```python
from build123d import *

# Parameters (mm, degrees)
SKETCH_1_W               = 23
SKETCH_1_H               = 27.6
SKETCH_1_W_2             = 4.5
SKETCH_1_H_2             = 1.2
EXTRUDE_1_DEPTH          = 6
SKETCH_2_R               = 4.2
EXTRUDE_2_DEPTH          = 0.85
CHAMFER_1_SIZE           = 0.3
SKETCH_4_R               = 2.5
SKETCH_4_R_2             = 1
EXTRUDE_3_DEPTH          = 3
CUT_EXTRUDE_1_DEPTH      = 28.699097458
CUT_EXTRUDE_1_DEPTH_BACK = 28.699097458
SKETCH_3_R               = 1.25
FILLET_1_R               = 1
SKETCH_5_W               = 5.6
SKETCH_5_H               = 3.5
EXTRUDE_4_DEPTH          = 3.5
SKETCH_6_R               = 0.6
EXTRUDE_7_DEPTH          = 6.5


with BuildPart() as part:
    # Эскиз1 → Бобышка-Вытянуть1 (new, symmetric)
    with BuildSketch(Plane.XY):
        Rectangle(SKETCH_1_W, SKETCH_1_H)
        with Locations((-13.75, 7.4)):
            Rectangle(SKETCH_1_W_2, SKETCH_1_H_2)
        with Locations((13.75, 7.4)):
            Rectangle(SKETCH_1_W_2, SKETCH_1_H_2)
    extrude(amount=EXTRUDE_1_DEPTH, both=True)

    # Эскиз2 → Бобышка-Вытянуть2 (add)
    with BuildSketch(Plane(origin=(0, 13.8, 0), x_dir=(1, 0, 0), z_dir=(0, 1, 0))):
        with Locations(Location((-5.8, 0, 0), (0, 0, 270))):
            Circle(SKETCH_2_R)
    extrude(amount=EXTRUDE_2_DEPTH)

    # Фаска1
    chamfer_1_edges = [part.edges().sort_by_distance(p)[0] for p in [
        (-5.8, 14.65, -4.2),
    ]]
    chamfer(chamfer_1_edges, length=CHAMFER_1_SIZE)

    # Эскиз4 → Бобышка-Вытянуть3 (add)
    with BuildSketch(Plane(origin=(0, 14.65, 0), x_dir=(1, 0, 0), z_dir=(0, 1, 0))):
        with Locations(Location((-5.8, 0, 0), (0, 0, 270))):
            Circle(SKETCH_4_R)
        with Locations(Location((-5.8, 0, 0), (0, 0, 270))):
            Circle(SKETCH_4_R_2, mode=Mode.SUBTRACT)
    extrude(amount=EXTRUDE_3_DEPTH)

    # Эскиз3 → Вырез-Вытянуть1 (cut, two sides: drawn at the far end of the back side and taken through both)
    with BuildSketch(Plane(origin=(0, 8, 0), x_dir=(1, 0, 0), z_dir=(0, 1, 0)).offset(-CUT_EXTRUDE_1_DEPTH_BACK)):
        with Locations(Location((-13.75, 3.5, 0), (0, 0, 270))):
            Circle(SKETCH_3_R)
        with Locations(Location((-13.75, -3.5, 0), (0, 0, 270))):
            Circle(SKETCH_3_R)
        with Locations(Location((13.75, -3.5, 0), (0, 0, 90))):
            Circle(SKETCH_3_R)
        with Locations(Location((13.75, 3.5, 0), (0, 0, 90))):
            Circle(SKETCH_3_R)
        with BuildLine():
            Line((-16, 1.1), (-13.6, 1.1))
            ThreePointArc((-13.6, 1.1), (-12.5, 0), (-13.6, -1.1))
            Line((-13.6, -1.1), (-16, -1.1))
            Line((-16, -1.1), (-16, 1.1))
        make_face()
        with BuildLine():
            Line((16, 1.1), (13.6, 1.1))
            ThreePointArc((13.6, 1.1), (12.5, 0), (13.6, -1.1))
            Line((13.6, -1.1), (16, -1.1))
            Line((16, -1.1), (16, 1.1))
        make_face()
    extrude(amount=CUT_EXTRUDE_1_DEPTH + CUT_EXTRUDE_1_DEPTH_BACK, mode=Mode.SUBTRACT)

    # Скругление1
    fillet_1_edges = [part.edges().sort_by_distance(p)[0] for p in [
        (-16, 7.4, -6),
        (16, 7.4, -6),
        (16, 7.4, 6),
        (-16, 7.4, 6),
    ]]
    fillet(fillet_1_edges, radius=FILLET_1_R)

    # Эскиз5 → Бобышка-Вытянуть4 (add)
    with BuildSketch(Plane.ZY.offset(11.5)):
        with Locations((0, -6.65)):
            Rectangle(SKETCH_5_W, SKETCH_5_H)
    extrude(amount=EXTRUDE_4_DEPTH)

    # Эскиз6 → Бобышка-Вытянуть7 (add)
    with BuildSketch(Plane.ZY.offset(15)):
        with Locations((0, -6.65)):
            Circle(SKETCH_6_R)
        with Locations(Location((1.3, -6.65, 0), (0, 0, 180))):
            Circle(SKETCH_6_R)
        with Locations(Location((-1.3, -6.65, 0), (0, 0, 180))):
            Circle(SKETCH_6_R)
    extrude(amount=EXTRUDE_7_DEPTH)


solid = part.part
```
The model under review builds one solid part; all positions refer to its coordinate system, in mm. A direction names the side the tool comes from. Coordinates: 2 decimals unless noted, no trailing zeros. Order: outer loops, then holes, each group sorted by start corner. A loop starts at its lowest first (then second) coordinate and runs counter-clockwise, first axis right, second up. Notation, with made-up numbers: (37, 78.25) -> (78, 78.25) arc R21 ccw to (78, 104.25) -> close; hole circle Ø3 at (17, 43). An arc over 180 degrees is marked (long way). Answer in a Markdown table with one row per item. Add a question column.
Item 1: Machinability: for faces 4 (the cylindrical face through (-6.776, 16.129, -0.217)), 5 (the flat face through (-13, -7, -2.8)), 6 (the flat face through (-11.5, 11, 0)), which of the approach directions +Z, -Z, +X, -X, +Y, -Y give a long, thin tool a straight path to every point of the face, cutting with its end or side? Answer none if there is none.
Item 2: Clearance check with flat-ended pins moving along their axes: pin 1 (5 mm diameter, centred on x = -12, z = 0, fed in from +Y); pin 2 (2 mm diameter, centred on x = -14, z = 4, fed in from -Y); pin 3 (1 mm diameter, centred on x = -12.5, y = -7, fed in from +Z). State where each tip first meets the part, or that it passes through.
Item 3: Mouldability with a two-part tool opening along Z and no side actions: class faces 1 (the flat face through (-15, 7, -1.1)), 2 (the flat face through (11.5, -4, 0)), 3 (the cylindrical face through (-15.699, 7.408, 5.715)) as +Z half, -Z half, draft (parallel to the pull), parting line (faces both ways), or undercut.
Item 4: We need section C-C on y = -3.5. Write out the cut boundary in (x, z).
Item 5: We need section A-A on y = -6.65. Write out the cut boundary in (x, z), plus the area to 3 significant figures.
Item 6: We need section B-B on x = -5.8. Write out the cut boundary in (y, z).
Item 7: To check wall thickness, follow probe 1 along X at (y, z) = (7.75, 3.5); probe 2 along Y at (x, z) = (6, 5); probe 3 along X at (y, z) = (16.8, 0). State the ranges of each line that lie inside material, in increasing order.
Final values:
| question | item | result |
|---|---|---|
| 1 | face 4 | +Y |
| 1 | face 5 | -Z, -X, -Y |
| 1 | face 6 | +Z, -Z, -X, +Y |
| 2 | pin 1 | stops at y = 14.65 |
| 2 | pin 2 | stops at y = 6.8 |
| 2 | pin 3 | stops at z = 2.8 |
| 3 | face 1 | undercut |
| 3 | face 2 | draft |
| 3 | face 3 | +Z half |
| 4 | outline | (-11.5, -6) -> (11.5, -6) -> (11.5, 6) -> (-11.5, 6) -> close |
| 5 | outline | (-21.5, -1.9) -> (-15, -1.9) -> (-15, -2.8) -> (-11.5, -2.8) -> (-11.5, -6) -> (11.5, -6) -> (11.5, 6) -> (-11.5, 6) -> (-11.5, 2.8) -> (-15, 2.8) -> (-15, 1.9) -> (-21.5, 1.9) -> (-21.5, 0.7) -> (-15, 0.7) -> (-15, 0.6) -> (-21.5, 0.6) -> (-21.5, -0.6) -> (-15, -0.6) -> (-15, -0.7) -> (-21.5, -0.7) -> close |
| 5 | area | 319 mm2 |
| 6 | outline | (-13.8, -6) -> (13.8, -6) -> (13.8, -4.2) -> (14.35, -4.2) -> (14.65, -3.9) -> (14.65, -2.5) -> (17.65, -2.5) -> (17.65, -1) -> (14.65, -1) -> (14.65, 1) -> (17.65, 1) -> (17.65, 2.5) -> (14.65, 2.5) -> (14.65, 3.9) -> (14.35, 4.2) -> (13.8, 4.2) -> (13.8, 6) -> (-13.8, 6) -> close |
| 7 | probe 1 | x = -16 to -15, -12.5 to 12.5, 15 to 16 |
| 7 | probe 2 | y = -13.8 to 13.8 |
| 7 | probe 3 | x = -8.3 to -6.8, -4.8 to -3.3 |
